```python
from build123d import *

# Parameters (mm, degrees)
SKETCH1_R           = 1.8
BOSS_EXTRUDE1_DEPTH = 13
SKETCH2_R           = 4
CUT_EXTRUDE1_DEPTH  = 10
SKETCH3_R           = 11.75
CUT_EXTRUDE2_DEPTH  = 4.5
SKETCH4_R           = 6
CUT_EXTRUDE3_DEPTH  = 6.5
CUT_EXTRUDE6_DEPTH  = 45.606330279
FILLET1_R           = 5


with BuildPart() as part:
    # Sketch1 → Boss-Extrude1 (new, symmetric)
    with BuildSketch(Plane(origin=(0, 0, 0), x_dir=(0, 0, -1), z_dir=(1, 0, 0))):
        with BuildLine():
            Line((0, 0), (0, 40))
            Line((0, 40), (-12, 40))
            Line((-12, 40), (-12, 5.5))
            ThreePointArc((-12, 5.5), (-14.374806505, -1.183390223), (-7.70361619, -3.592255225))
            Line((-7.70361619, -3.592255225), (0, 0))
        make_face()
        with Locations(Location((-9.828619755, 0.964829626, 0), (0, 0, 180))):
            Circle(SKETCH1_R, mode=Mode.SUBTRACT)
    extrude(amount=BOSS_EXTRUDE1_DEPTH, both=True)

    # Sketch2 → Cut-Extrude1 (cut, symmetric)
    with BuildSketch(Plane(origin=(0, 0, 0), x_dir=(0, 0, -1), z_dir=(1, 0, 0))):
        with Locations((-9.5, 19)):
            Circle(SKETCH2_R)
    extrude(amount=CUT_EXTRUDE1_DEPTH, both=True, mode=Mode.SUBTRACT)

    # Sketch3 → Cut-Extrude2 (cut, symmetric)
    with BuildSketch(Plane(origin=(0, 0, 0), x_dir=(0, 0, -1), z_dir=(1, 0, 0))):
        with Locations((-9.5, 19)):
            Circle(SKETCH3_R)
    extrude(amount=CUT_EXTRUDE2_DEPTH, both=True, mode=Mode.SUBTRACT)

    # Sketch4 → Cut-Extrude3 (cut, symmetric)
    with BuildSketch(Plane(origin=(0, 0, 0), x_dir=(0, 0, -1), z_dir=(1, 0, 0))):
        with Locations((-9.828619755, 0.964829626)):
            Circle(SKETCH4_R)
    extrude(amount=CUT_EXTRUDE3_DEPTH, both=True, mode=Mode.SUBTRACT)

    # Sketch7 → Cut-Extrude6 (cut, through all)
    with BuildSketch(Plane(origin=(0, 0, 0), x_dir=(-1, 0, 0), z_dir=(0, 0, -1))):
        with BuildLine():
            Line((-6.25, 35.75), (-6.25, 33.75))
            ThreePointArc((-6.25, 33.75), (-8, 32), (-9.75, 33.75))
            Line((-9.75, 33.75), (-9.75, 35.75))
            ThreePointArc((-9.75, 35.75), (-8, 37.5), (-6.25, 35.75))
        make_face()
        with BuildLine():
            Line((9.75, 35.75), (9.75, 33.75))
            ThreePointArc((9.75, 33.75), (8, 32), (6.25, 33.75))
            Line((6.25, 33.75), (6.25, 35.75))
            ThreePointArc((6.25, 35.75), (8, 37.5), (9.75, 35.75))
        make_face()
    extrude(amount=-CUT_EXTRUDE6_DEPTH, mode=Mode.SUBTRACT)

    # Fillet1
    fillet1_edges = [part.edges().sort_by_distance(p)[0] for p in [
        (13, 40, 6),
        (-13, 40, 6),
    ]]
    fillet(fillet1_edges, radius=FILLET1_R)


solid = part.part
```
Geometry: final body of the model. Coordinates: model frame, mm. A direction names the side the tool comes from. Round coordinates to 2 decimals unless told otherwise and drop trailing zeros. Loops run counter-clockwise (first coordinate to the right, second up) from the corner with the lowest first, then second, coordinate; pieces in that order, holes last.
Item 1: Mould query, pull axis Z, two halves, no side actions, for faces 1 (the cylindrical face through (-9.704, -1.083, 14.421)), 2 (the flat face through (9.75, 35, 6)), 3 (the cylindrical face through (0.063, 29.948, 5.232)). Classes: released by +Z, released by -Z, zero draft, split by the parting line, or undercut.
Checked values:
face 1: split by the parting line
face 2: zero draft
face 3: undercut
Item 2: Section D-D, the plane z = 1.5. Output: boundary loops of the cut face in (x, y).
Checked values:
outline: (-13, -0.7) - (13, -0.7) - (13, 35) arc R5 ccw to (8, 40) - (-8, 40) arc R5 ccw to (-13, 35) - close; hole (-9.75, 33.75) arc R1.75 ccw to (-6.25, 33.75) - (-6.25, 35.75) arc R1.75 ccw to (-9.75, 35.75) - close; hole (-4.5, 10.39) - (4.5, 10.39) - (4.5, 27.61) - (-4.5, 27.61) - close; hole (6.25, 33.75) arc R1.75 ccw to (9.75, 33.75) - (9.75, 35.75) arc R1.75 ccw to (6.25, 35.75) - close
Item 3: Reachability of faces 4 (the flat face through (-6, 23, 12)), 5 (the cylindrical face through (-8, 32, 6)), 6 (the flat face through (6, 20, 0)), 7 (the cylindrical face through (7.3, 18.9, 5.5)), 8 (the flat face through (13, 16, 6)) from +Z, -Z, +X, -X, +Y, -Y: full face, straight path, thin tool, end or side. Return the list, or none.
Checked values:
face 4: +Z, +X, -X, +Y
face 5: +Z, -Z
face 6: -Z, +X, -X, +Y, -Y
face 7: none
face 8: +Z, -Z, +X, +Y, -Y
Item 4: Section C-C, the plane x = 2.5. Output: boundary loops of the cut face in (y, z), plus the area to 3 significant figures.
Checked values:
outline: (-2.21, 4.74) - (0, 0) - (12.09, 0) arc R11.75 cw to (7.52, 12) - (6.56, 12) arc R6 cw to start; (25.91, 0) - (40, 0) - (40, 12) - (30.48, 12) arc R11.75 cw to start
area: 181 mm2
Item 5: Line query: L1, parallel to X at y = 35, z = 10; L2, parallel to X at y = 10, z = 2.25; L3, parallel to Y at x = -9, z = 11.25. Output: solid intervals per line, ascending.
Checked values:
L1: x = -13 to -9.75, -6.25 to 6.25, 9.75 to 13
L2: x = -13 to -4.5, 4.5 to 13
L3: y = -3.86 to -0.14, 2.07 to 15.4, 22.6 to 32.31, 37.19 to 39.9
Item 6: Contact query for flat-ended pins moving along their axis: P1, Ø5.5, axis at y = 0, z = 11, coming from the -X side; P2, Ø1, axis at x = 0, z = 4, coming from the -Y side; P3, Ø2, axis at x = 4, y = 34.5, coming from the +Z side. Output: stop coordinate, or through.
Checked values:
P1: stops at x = -13
P2: stops at y = -2.1
P3: stops at z = 12
Item 7: Section B-B, the plane z = 12.5. Output: boundary loops of the cut face in (x, y).
Checked values:
outline: (-13, -3.3) - (-6.5, -3.3) - (-6.5, 5.22) - (-13, 5.22) - close; (6.5, -3.3) - (13, -3.3) - (13, 5.22) - (6.5, 5.22) - close
Item 8: Section A-A, the plane y = 19. Output: boundary loops of the cut face in (x, z).
Checked values:
outline: (-13, 0) - (-4.5, 0) - (-4.5, 5.5) - (-10, 5.5) - (-10, 12) - (-13, 12) - close; (4.5, 0) - (13, 0) - (13, 12) - (10, 12) - (10, 5.5) - (4.5, 5.5) - close
